Geometry: final body of the model. Coordinates: model frame, mm. Face numbers are marked on the shaded views. A direction names the side the tool comes from. Give positions to 0.01 mm unless a question says otherwise; leave off trailing zeros. Write each loop counter-clockwise with the first axis right and the second up, starting at its lowest first coordinate (ties: lowest second). Pieces come first, ordered by that corner, then holes. Notation, with made-up numbers: M 75,14.25 L 123,14.25 A11 ccw 123,26.25 Z; hole C -24.75,35 d4. An arc over 180 degrees is marked long. Use a Markdown table: item, result. Add a question column.
1) Pin query (flat end, axial travel): pin 1 (5 mm diameter, centred on x = 24, y = 37, fed in from +Z); pin 2 (6 mm diameter, centred on x = 44.5, y = 47.5, fed in from +Z). Return the tip coordinate at first contact, or that it passes through.
2) Set-up query: the marked faces 1 and 2. Return all of +Z, -Z, +X, -X, +Y, -Y with unobstructed straight access to the full face (end or side cutting, diameter ignored); none if empty.
3) Line query: line 1 (X direction, y = 10.5, z = 8.5); line 2 (Z direction, x = -36.5, y = -22.5). Output: solid intervals per line, ascending.
4) Draft query along Y for the marked faces 3, 4 and 5. Return one class per face: +Y half, -Y half, draft (parallel to the pull), parting line (faces both ways), or undercut.
5) Section A-A on x = -34. Return the cut outline in (y, z).
```python
from build123d import *

# Parameters (mm, degrees)
F1_DEPTH      = 15
F3_DEPTH      = 10
F5_R          = 5
F6_DEPTH      = 15
F8_R          = 5
F9_DEPTH      = 15
F11_R         = 5
F12_DEPTH     = 15
F14_R         = 5
F15_DEPTH     = 15
F16_T1_DEPTH  = 32.443405813
F16_T3_DEPTH  = 32.443405813
F16_T5_DEPTH  = 32.443405813
F16_T7_DEPTH  = 32.443405813
F16_T9_DEPTH  = 32.443405813
F16_T11_DEPTH = 32.443405813
F16_T13_DEPTH = 32.443405813
F16_T15_DEPTH = 32.443405813
F17_R         = 5
F18_R         = 5


# Not quite as in the source:
# - a fillet or chamfer that OpenCascade refuses, or shapes differently, is made with other operations: its cross-section is extruded or revolved along the edge and cut away or added


with BuildPart() as f1:
    # F0 (on Top) → F1 (new body)
    with BuildSketch(Plane.XY):
        Polygon((50, 60), (-50, 60), (-60, 50), (-60, -50), (-50, -60), (50, -60), (60, -50), (60, 50), align=None)
    extrude(amount=F1_DEPTH)

    # F2 (on face) → F3 (cut)
    with BuildSketch(Plane.XY.offset(15)):
        Polygon((40, 50), (-40, 50), (-50, 40), (-50, -40), (-40, -50), (40, -50), (50, -40), (50, 40), align=None)
    extrude(amount=-F3_DEPTH, mode=Mode.SUBTRACT)

    # F5 (on offset) → F6 (cut)
    with BuildSketch(Plane(origin=(-55.0707106781, 55.0707106781, 0), x_dir=(-0.7071067812, -0.7071067812, 0), z_dir=(-0.7071067812, 0.7071067812, 0))):
        with Locations((0, 15)):
            Circle(F5_R)
    extrude(amount=-F6_DEPTH, mode=Mode.SUBTRACT)

    # F8 (on offset) → F9 (cut)
    with BuildSketch(Plane(origin=(55.0707106781, 55.0707106781, 0), x_dir=(-0.7071067812, 0.7071067812, 0), z_dir=(0.7071067812, 0.7071067812, 0))):
        with Locations((0, 15)):
            Circle(F8_R)
    extrude(amount=-F9_DEPTH, mode=Mode.SUBTRACT)

    # F11 (on offset) → F12 (cut)
    with BuildSketch(Plane(origin=(55.0707106781, -55.0707106781, 0), x_dir=(0.7071067812, 0.7071067812, 0), z_dir=(0.7071067812, -0.7071067812, 0))):
        with Locations((0, 15)):
            Circle(F11_R)
    extrude(amount=-F12_DEPTH, mode=Mode.SUBTRACT)

    # F14 (on offset) → F15 (cut)
    with BuildSketch(Plane(origin=(-55.0707106781, -55.0707106781, 0), x_dir=(0.7071067812, -0.7071067812, 0), z_dir=(-0.7071067812, -0.7071067812, 0))):
        with Locations((0, 15)):
            Circle(F14_R)
    extrude(amount=-F15_DEPTH, mode=Mode.SUBTRACT)

    # F16: fillet of radius 5 on 8 edges, made by hand

    # F16_s2 → F16_t1 (cut)
    with BuildSketch(Plane(origin=(-61.4704761276, 61.4704761276, 0), x_dir=(0, 0, 1), z_dir=(0.7071067812, -0.7071067812, 0))):
        with BuildLine():
            ThreePointArc((15, 8.6602540378), (14.3301270189, 6.1602540378), (12.5, 4.3301270189))
            ThreePointArc((12.5, 4.3301270189), (13.7059047745, 4.8296291314), (15, 5))
            Line((15, 5), (15, 8.6602540378))
        make_face()
    extrude(amount=F16_T1_DEPTH, mode=Mode.SUBTRACT)

    # F16_s4 → F16_t3 (cut)
    with BuildSketch(Plane(origin=(-38.5295238724, 38.5295238724, 0), x_dir=(0, 0, 1), z_dir=(-0.7071067812, 0.7071067812, 0))):
        with BuildLine():
            ThreePointArc((15, 8.6602540378), (14.3301270189, 6.1602540378), (12.5, 4.3301270189))
            ThreePointArc((12.5, 4.3301270189), (13.7059047745, 4.8296291314), (15, 5))
            Line((15, 5), (15, 8.6602540378))
        make_face()
    extrude(amount=F16_T3_DEPTH, mode=Mode.SUBTRACT)

    # F16_s6 → F16_t5 (cut)
    with BuildSketch(Plane(origin=(-38.5295238724, -38.5295238724, 0), x_dir=(0, 0, 1), z_dir=(-0.7071067812, -0.7071067812, 0))):
        with BuildLine():
            ThreePointArc((15, 8.6602540378), (14.3301270189, 6.1602540378), (12.5, 4.3301270189))
            ThreePointArc((12.5, 4.3301270189), (13.7059047745, 4.8296291314), (15, 5))
            Line((15, 5), (15, 8.6602540378))
        make_face()
    extrude(amount=F16_T5_DEPTH, mode=Mode.SUBTRACT)

    # F16_s8 → F16_t7 (cut)
    with BuildSketch(Plane(origin=(-61.4704761276, -61.4704761276, 0), x_dir=(0, 0, 1), z_dir=(0.7071067812, 0.7071067812, 0))):
        with BuildLine():
            ThreePointArc((12.5, 4.3301270189), (14.3301270189, 6.1602540378), (15, 8.6602540378))
            Line((15, 8.6602540378), (15, 5))
            ThreePointArc((15, 5), (13.7059047745, 4.8296291314), (12.5, 4.3301270189))
        make_face()
    extrude(amount=F16_T7_DEPTH, mode=Mode.SUBTRACT)

    # F16_s10 → F16_t9 (cut)
    with BuildSketch(Plane(origin=(61.4704761276, -61.4704761276, 0), x_dir=(0, 0, 1), z_dir=(-0.7071067812, 0.7071067812, 0))):
        with BuildLine():
            ThreePointArc((15, 8.6602540378), (14.3301270189, 6.1602540378), (12.5, 4.3301270189))
            ThreePointArc((12.5, 4.3301270189), (13.7059047745, 4.8296291314), (15, 5))
            Line((15, 5), (15, 8.6602540378))
        make_face()
    extrude(amount=F16_T9_DEPTH, mode=Mode.SUBTRACT)

    # F16_s12 → F16_t11 (cut)
    with BuildSketch(Plane(origin=(38.5295238724, -38.5295238724, 0), x_dir=(0, 0, 1), z_dir=(0.7071067812, -0.7071067812, 0))):
        with BuildLine():
            ThreePointArc((12.5, 4.3301270189), (14.3301270189, 6.1602540378), (15, 8.6602540378))
            Line((15, 8.6602540378), (15, 5))
            ThreePointArc((15, 5), (13.7059047745, 4.8296291314), (12.5, 4.3301270189))
        make_face()
    extrude(amount=F16_T11_DEPTH, mode=Mode.SUBTRACT)

    # F16_s14 → F16_t13 (cut)
    with BuildSketch(Plane(origin=(61.4704761276, 61.4704761276, 0), x_dir=(0, 0, 1), z_dir=(-0.7071067812, -0.7071067812, 0))):
        with BuildLine():
            ThreePointArc((15, 8.6602540378), (14.3301270189, 6.1602540378), (12.5, 4.3301270189))
            ThreePointArc((12.5, 4.3301270189), (13.7059047745, 4.8296291314), (15, 5))
            Line((15, 5), (15, 8.6602540378))
        make_face()
    extrude(amount=F16_T13_DEPTH, mode=Mode.SUBTRACT)

    # F16_s16 → F16_t15 (cut)
    with BuildSketch(Plane(origin=(38.5295238724, 38.5295238724, 0), x_dir=(0, 0, 1), z_dir=(0.7071067812, 0.7071067812, 0))):
        with BuildLine():
            ThreePointArc((12.5, 4.3301270189), (14.3301270189, 6.1602540378), (15, 8.6602540378))
            Line((15, 8.6602540378), (15, 5))
            ThreePointArc((15, 5), (13.7059047745, 4.8296291314), (12.5, 4.3301270189))
        make_face()
    extrude(amount=F16_T15_DEPTH, mode=Mode.SUBTRACT)

    # F17
    f17_edges = [f1.edges().sort_by_distance(p)[0] for p in [
        (-60, 50, 7.370363),
        (-50, 60, 7.370363),
        (-60, -50, 7.370363),
        (-50, -60, 7.370363),
        (50, -60, 7.370363),
        (60, -50, 7.370363),
        (60, 50, 7.370363),
        (50, 60, 7.370363),
    ]]
    fillet(f17_edges, radius=F17_R)

    # F18
    f18_edges = [f1.edges().sort_by_distance(p)[0] for p in [
        (-40, -50, 9.870363),
        (-50, -40, 9.870363),
        (-50, 40, 9.870363),
        (-40, 50, 9.870363),
        (40, 50, 9.870363),
        (50, 40, 9.870363),
        (50, -40, 9.870363),
        (40, -50, 9.870363),
    ]]
    fillet(f18_edges, radius=F18_R)


solid = f1.part
```
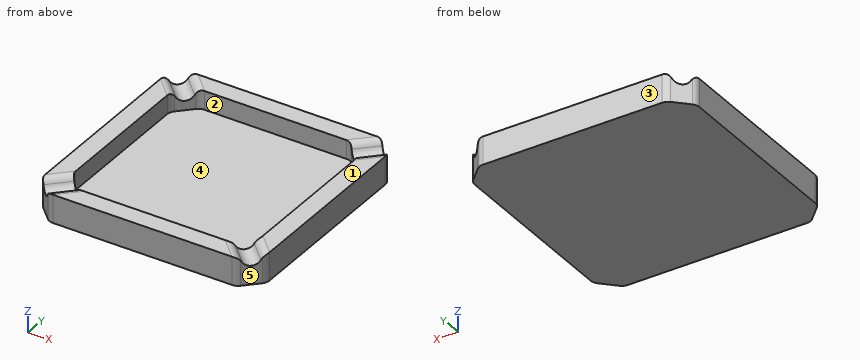
Found:
| question | item | result |
|---|---|---|
| 1 | pin 1 | z = 5 |
| 1 | pin 2 | z = 13.53 |
| 2 | face 1 | +Z, +X, -X, +Y, -Y |
| 2 | face 2 | +Z |
| 3 | line 1 | -60 to -50, 50 to 60 |
| 3 | line 2 | 0 to 5 |
| 4 | face 3 | +Y half |
| 4 | face 4 | undercut |
| 4 | face 5 | -Y half |
| 5 | outline | M -60,0 L 60,0 L 60,15 L 50,15 L 50,5 L -50,5 L -50,15 L -60,15 Z |
